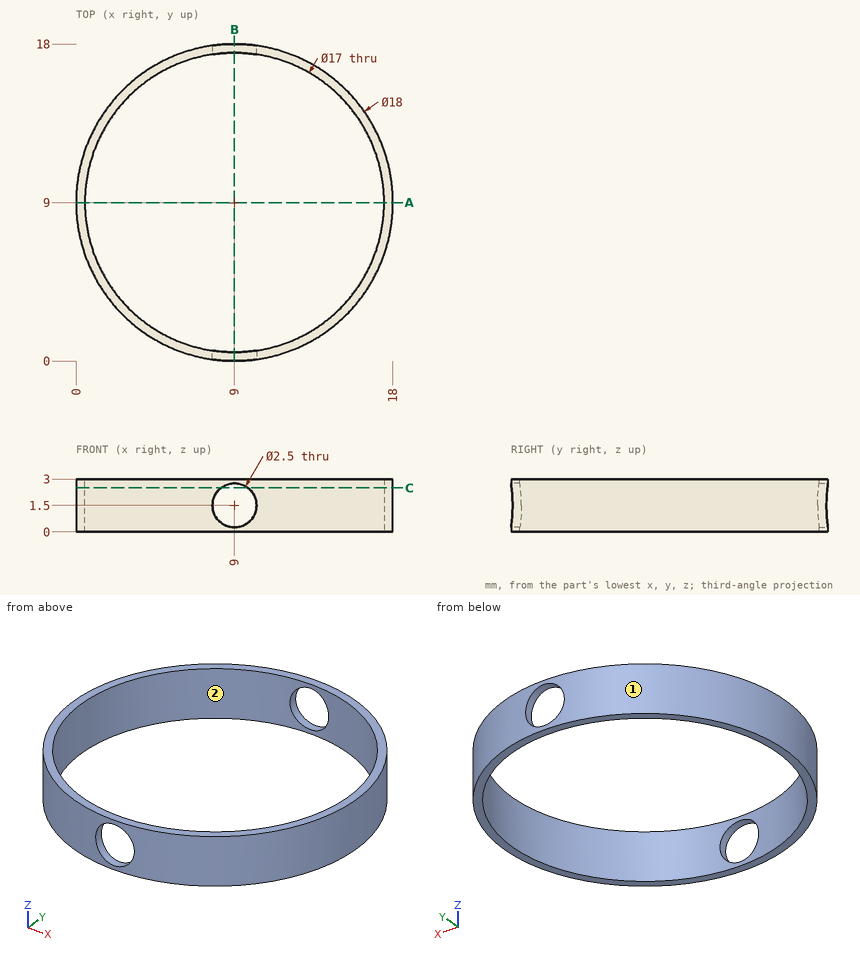
Could you check a few things on this drawing? It's one solid part, dimensions in mm from its lowest x, y, z. Coordinates: 2 decimals unless noted, no trailing zeros. Write each loop counter-clockwise with the first axis right and the second up, starting at its lowest first coordinate (ties: lowest second). Pieces come first, ordered by that corner, then holes. Notation, with made-up numbers: (62, 40.5) - (97, 40.5) arc R26 cw to (97, 66.5) - close; hole circle Ø1 at (-2, 46.25). An arc over 180 degrees is marked (long way). Put each result on its own line as item: value. Start each with the question number.
Q1. I want a section at A-A on y = 9. Write out the boundary of the cut face in (x, z).
Q2. I want a section at C-C on z = 2.5. Write out the boundary of the cut face in (x, y).
Q3. Please list where these lines run through material, in increasing order: L1, parallel to Z at x = 9, y = 17.65; L2, parallel to X at y = 9.25, z = 1.35; L3, parallel to Y at x = 1.5, z = 1.4.
Q4. Thinking about a two-plate mould opening in Y: for the marked faces 1 and 2, which applies, pulls with the +Y half, pulls with the -Y half, needs draft (parallel to the pull), parting line crosses it, or undercut?
Q5. I want a section at B-B on x = 9. Write out the boundary of the cut face in (y, z).
Q6. I'm going to push flat-ended pins straight in: P1, Ø1.5, axis at x = 12.5, z = 1, coming from the +Y side; P2, Ø1.5, axis at y = 6.5, z = 2, coming from the +X side; P3, Ø1, axis at y = 7.5, z = 1.5, coming from the +X side. Where does each tip first touch, or does it pass through?
Checks:
1. outline: (0, 0) - (0.5, 0) - (0.5, 3) - (0, 3) - close; (17.5, 0) - (18, 0) - (18, 3) - (17.5, 3) - close
2. outline: (8.25, 0.03) - (8.25, 0.53) arc R8.5 cw to (8.25, 17.47) - (8.25, 17.97) arc R9 ccw to start; (9.75, 0.03) arc R9 ccw to (9.75, 17.97) - (9.75, 17.47) arc R8.5 cw to (9.75, 0.53) - close
3. L1: 0 to 0.25, 2.75 to 3
3. L2: 0 to 0.5, 17.5 to 18
3. L3: 4.03 to 5, 13 to 13.97
4. face 1: parting line crosses it
4. face 2: undercut
5. outline: (0, 0) - (0.5, 0) - (0.5, 0.25) - (0, 0.25) - close; (0, 2.75) - (0.5, 2.75) - (0.5, 3) - (0, 3) - close; (17.5, 0) - (18, 0) - (18, 0.25) - (17.5, 0.25) - close; (17.5, 2.75) - (18, 2.75) - (18, 3) - (17.5, 3) - close
6. P1: y = 17.57
6. P2: x = 17.83
6. P3: x = 17.94
